Design review of the part built by this model. Coordinates are the model's own, in mm. A direction names the side the tool comes from. Coordinates: 2 decimals unless noted, no trailing zeros. Order: outer loops, then holes, each group sorted by start corner. A loop starts at its lowest first (then second) coordinate and runs counter-clockwise, first axis right, second up. Notation, with made-up numbers: (88, -1.5) -> (147, -1.5) arc R29 cw to (147, 20.5) -> close; hole circle Ø7 at (-31, -27.5). An arc over 180 degrees is marked (long way). Write item = value, one per line.
```python
from build123d import *

# Parameters (mm, degrees)
SKETCH001_W  = 2.9
SKETCH001_H  = 2.9
POCKET_DEPTH = 3
CHAMFER_SIZE = 0.2


with BuildPart() as part:
    # Sketch → Revolution (revolve)
    with BuildSketch(Plane.XZ):
        Polygon((0, 9), (2.5, 9), (2.5, 6), (3, 6), (3, 0), (0, 0), align=None)
    revolve(axis=Axis((0, 0, 0), (0, 0, 1)))

    # Sketch001 (on Face5 of Revolution) → Pocket (cut)
    with BuildSketch(Plane(origin=(0, 0, 0), x_dir=(1, 0, 0), z_dir=(0, 0, -1))):
        Rectangle(SKETCH001_W, SKETCH001_H)
    extrude(amount=-POCKET_DEPTH, mode=Mode.SUBTRACT)

    # Chamfer
    chamfer_edges = [part.edges().sort_by_distance(p)[0] for p in [
        (-2.5, 0, 9),
    ]]
    chamfer(chamfer_edges, length=CHAMFER_SIZE)


solid = part.part
```
(1) We need section C-C (z = 1). Write out the cut boundary in (x, y).
Report:
outline = circle Ø6 at (0, 0); hole (-1.45, -1.45) -> (1.45, -1.45) -> (1.45, 1.45) -> (-1.45, 1.45) -> close
(2) We need section D-D (z = 4.5). Write out the cut boundary in (x, y).
Report:
outline = circle Ø6 at (0, 0)
(3) For L1, parallel to Z at x = -1.95, y = -2; L2, parallel to Z at x = 1, y = -0.35; L3, parallel to Y at x = 0.1, z = 6.75, list the stretches that pass through material, from the lowest coordinate up.
Report:
L1 = 0 to 6
L2 = 3 to 9
L3 = -2.5 to 2.5
(4) The part is to be moulded in two halves that separate along X. For faces 4 (the flat face through (2, 2, 6)), 5 (the flat face through (1.45, 0, 1)), 6 (the cylindrical face through (-3, 0, 3)), 7 (the flat face through (0, 0, 3)), say which applies: released by +X, released by -X, zero draft, split by the parting line, or undercut.
Report:
face_4 = zero draft
face_5 = undercut
face_6 = split by the parting line
face_7 = undercut
(5) We need section A-A (x = 0). Write out the cut boundary in (y, z), and give its area (3 significant figures).
Report:
outline = (-3, 0) -> (-1.45, 0) -> (-1.45, 3) -> (1.45, 3) -> (1.45, 0) -> (3, 0) -> (3, 6) -> (2.5, 6) -> (2.5, 8.8) -> (2.3, 9) -> (-2.3, 9) -> (-2.5, 8.8) -> (-2.5, 6) -> (-3, 6) -> close
area = 42.3 mm²
(6) For faces 1 (the flat face through (0, -2, 0)), 2 (the cylindrical face through (-0.54, -2.44, 7.38)), 3 (the flat face through (0, 1.45, 1)), list the 3-axis set-ups (+Z, -Z, +X, -X, +Y, -Y) from which the entire face can be reached by the end or side of a thin tool; tool diameter is ignored.
Report:
face_1 = -Z, +X, -X, +Y, -Y
face_2 = +Z
face_3 = -Z
(7) Insertion check: pin 1 (2 mm diameter, centred on y = -2, z = 1, fed in from +X); pin 2 (1 mm diameter, centred on y = -1.5, z = 1, fed in from -X). Each pin has a flat end and moves straight along its axis. Give the tip position at first contact, or say it passes through.
Report:
pin_1 = 2.83
pin_2 = -2.83
